Input: part model. Units: mm. Frame: model coordinates. Face numbers are marked on the shaded views. A direction names the side the tool comes from. Coordinates: 2 decimals unless noted, no trailing zeros. Loops run counter-clockwise (first coordinate to the right, second up) from the corner with the lowest first, then second, coordinate; pieces in that order, holes last.
```python
from build123d import *

# Parameters (mm, degrees)
SKETCH1_R           = 1.143
SKETCH1_R_2         = 0.6985
BOSS_EXTRUDE1_DEPTH = 2.54


with BuildPart() as part:
    # Sketch1 → Boss-Extrude1 (new body)
    with BuildSketch(Plane.XY):
        with BuildLine():
            Line((-2.544193385, 2.54), (-2.544193385, -1.524))
            ThreePointArc((-2.544193385, -1.524), (-2.246613875, -2.24242049), (-1.528193385, -2.54))
            Line((-1.528193385, -2.54), (6.599806615, -2.54))
            ThreePointArc((6.599806615, -2.54), (7.318227104, -2.83757951), (7.615806615, -3.556))
            Line((7.615806615, -3.556), (7.615806615, -9.91))
            ThreePointArc((7.615806615, -9.91), (12.695806615, -14.99), (17.775806615, -9.91))
            Line((17.775806615, -9.91), (17.775806615, -3.556))
            ThreePointArc((17.775806615, -3.556), (18.073386125, -2.83757951), (18.791806615, -2.54))
            Line((18.791806615, -2.54), (26.919806615, -2.54))
            ThreePointArc((26.919806615, -2.54), (27.638227104, -2.24242049), (27.935806615, -1.524))
            Line((27.935806615, -1.524), (27.935806615, 2.54))
            ThreePointArc((27.935806615, 2.54), (26.447909063, 6.132102448), (22.855806615, 7.62))
            Line((22.855806615, 7.62), (2.535806615, 7.62))
            ThreePointArc((2.535806615, 7.62), (-1.056295834, 6.132102448), (-2.544193385, 2.54))
        make_face()
        with Locations(Location((2.535806615, 2.54, 0), (0, 0, 180))):
            Circle(SKETCH1_R, mode=Mode.SUBTRACT)
        with Locations(Location((12.695806615, -9.91, 0), (0, 0, 180))):
            Circle(SKETCH1_R_2, mode=Mode.SUBTRACT)
        with Locations(Location((22.855806615, 2.54, 0), (0, 0, 180))):
            Circle(SKETCH1_R, mode=Mode.SUBTRACT)
    extrude(amount=BOSS_EXTRUDE1_DEPTH)


solid = part.part
```
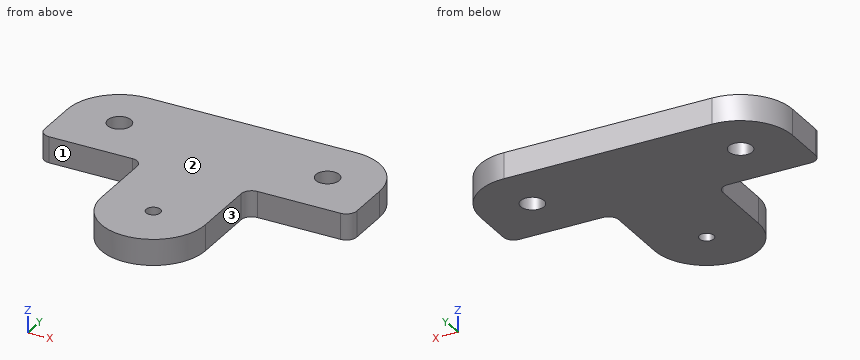
Item 1: Section query D-D (x = 26). Output: boundary loops of the cut face in (y, z), then the cut area to 3 significant figures.
Result:
outline: (-2.54, 0) - (6.53, 0) - (6.53, 2.54) - (-2.54, 2.54) - close
area: 23.0 mm2
Item 2: Section query B-B (x = 13). Output: boundary loops of the cut face in (y, z), then the cut area to 3 significant figures.
Result:
outline: (-14.98, 0) - (-10.54, 0) - (-10.54, 2.54) - (-14.98, 2.54) - close; (-9.28, 0) - (7.62, 0) - (7.62, 2.54) - (-9.28, 2.54) - close
area: 54.2 mm2
Item 3: Section query A-A (z = 1.3). Output: boundary loops of the cut face in (x, y).
Result:
outline: (-2.54, -1.52) arc R1.02 ccw to (-1.53, -2.54) - (6.6, -2.54) arc R1.02 cw to (7.62, -3.56) - (7.62, -9.91) arc R5.08 ccw to (17.78, -9.91) - (17.78, -3.56) arc R1.02 cw to (18.79, -2.54) - (26.92, -2.54) arc R1.02 ccw to (27.94, -1.52) - (27.94, 2.54) arc R5.08 ccw to (22.86, 7.62) - (2.54, 7.62) arc R5.08 ccw to (-2.54, 2.54) - close; hole circle Ø2.29 at (2.54, 2.54); hole circle Ø1.4 at (12.7, -9.91); hole circle Ø2.29 at (22.86, 2.54)
Item 4: Contact query for a flat-ended pin moving along its axis: P1, Ø1.3, axis at x = 12.7, y = -9.91, coming from the -Z side. Output: stop coordinate, or through.
Result:
P1: passes through
Item 5: Section query C-C (y = -6). Output: boundary loops of the cut face in (x, z).
Result:
outline: (7.62, 0) - (17.78, 0) - (17.78, 2.54) - (7.62, 2.54) - close
Item 6: Reachability of the marked faces 1, 2 and 3 from +Z, -Z, +X, -X, +Y, -Y: full face, straight path, thin tool, end or side. Return the list, or none.
Result:
face 1: +Z, -Z, -X, -Y
face 2: +Z, +X, -X, +Y, -Y
face 3: +Z, -Z, +X, -Y
Item 7: Line query: L1, parallel to X at y = 2.54, z = 1.3; L2, parallel to X at y = 2, z = 0.45; L3, parallel to Y at x = 5.5, z = 0.9. Output: solid intervals per line, ascending.
Result:
L1: x = -2.54 to 1.39, 3.68 to 21.71, 24 to 27.94
L2: x = -2.54 to 1.53, 3.54 to 21.85, 23.86 to 27.94
L3: y = -2.54 to 7.62
